Source: CAD feature listing. Evaluate the final solid. Frame: model axes, mm. Face numbers are marked on the shaded views. A direction names the side the tool comes from. Give positions to 0.01 mm unless a question says otherwise; leave off trailing zeros. Write each loop counter-clockwise with the first axis right and the second up, starting at its lowest first coordinate (ties: lowest second). Pieces come first, ordered by that corner, then holes. Notation, with made-up numbers: M 26,37.25 L 30,37.25 A15 ccw 30,41.25 Z; hole C 59.5,-1.5 d5. An arc over 180 degrees is marked long. Answer as a JSON object with one key per item and string values. Group by question number.
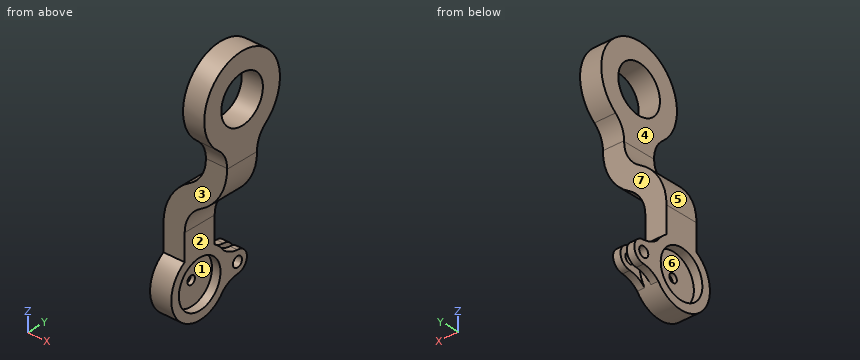
```python
from build123d import *

# Parameters (mm, degrees)
CROQUIS2_W              = 10
CROQUIS2_H              = 15.834903248
CROQUIS4_R              = 15
SALIENTE_EXTRUIR1_DEPTH = 10
CROQUIS5_R              = 20
SALIENTE_EXTRUIR2_DEPTH = 10
SALIENTE_EXTRUIR5_DEPTH = 3.5
CROQUIS13_R             = 2.4
CORTAR_EXTRUIR1_DEPTH   = 10
CROQUIS7_R              = 11
CORTAR_EXTRUIR3_DEPTH   = 10
REDONDEO2_R             = 12
REDONDEO3_R             = 12
CROQUIS14_R             = 11
CORTAR_EXTRUIR4_DEPTH   = 4
CROQUIS6_R              = 2
CORTAR_EXTRUIR5_DEPTH   = 6
CORTAR_EXTRUIR6_START   = -4
CROQUIS15_R             = 11
CORTAR_EXTRUIR6_DEPTH   = 4


with BuildPart() as part:
    # Barrer1: sweep along a path in Croquis1
    with BuildLine(Plane(origin=(0, 0, 0), x_dir=(1, 0, 0), z_dir=(0, 1, 0))) as barrer1_path:
        Line((-20, 85), (-20, 60))
        ThreePointArc((-20, 60), (-17.320508076, 50), (-10, 42.679491924))
        ThreePointArc((-10, 42.679491924), (-2.679491924, 35.358983849), (0, 25.358983849))
        Line((0, 25.358983849), (0, 0))
    # Croquis2 → Barrer1 (sweep)
    with BuildSketch(Plane.XY):
        Rectangle(CROQUIS2_W, CROQUIS2_H)
    sweep(path=barrer1_path.line)

    # Croquis4 → Saliente-Extruir1 (add)
    with BuildSketch(Plane(origin=(-15, 0, 0), x_dir=(0, 0, -1), z_dir=(1, 0, 0))):
        with Locations((85, 0)):
            Circle(CROQUIS4_R)
    extrude(amount=-SALIENTE_EXTRUIR1_DEPTH)

    # Croquis5 → Saliente-Extruir2 (add)
    with BuildSketch(Plane(origin=(5, 0, 0), x_dir=(0, 0, -1), z_dir=(1, 0, 0))):
        Circle(CROQUIS5_R)
    extrude(amount=-SALIENTE_EXTRUIR2_DEPTH)

    # Croquis12 → Saliente-Extruir5 (add)
    with BuildSketch(Plane(origin=(-15, 0, 0), x_dir=(0, 0, -1), z_dir=(1, 0, 0))):
        with BuildLine():
            ThreePointArc((90.068496439, 19.972615481), (85.068496439, 24.972615481), (80.068496439, 19.972615481))
            add(Edge.make_bspline(
                [(80.068496439, 19.972615481), (79.566731031, 15.028252388), (75.848465439, 11.643922813)],
                knots=[0, 0, 0, 1, 1, 1], degree=2))
            ThreePointArc((75.848465439, 11.643922813), (85.068496439, 14.846363713), (94.288527439, 11.643922813))
            add(Edge.make_bspline(
                [(90.068496439, 19.972615481), (90.570261847, 15.028252388), (94.288527439, 11.643922813)],
                knots=[0, 0, 0, 1, 1, 1], degree=2))
        make_face()
    saliente_extruir5 = extrude(amount=-SALIENTE_EXTRUIR5_DEPTH)

    # Simetría1: Saliente-Extruir5 across plane
    add(saliente_extruir5.mirror(Plane(origin=(-20, 0, 0), x_dir=(0, 0, 1), z_dir=(1, 0, 0))))

    # Croquis13 → Cortar-Extruir1 (cut)
    with BuildSketch(Plane(origin=(-15, 0, 0), x_dir=(0, 0, -1), z_dir=(1, 0, 0))):
        with Locations((85.068496439, 19.972615481)):
            Circle(CROQUIS13_R)
    extrude(amount=-CORTAR_EXTRUIR1_DEPTH, mode=Mode.SUBTRACT)

    # Croquis7 → Cortar-Extruir3 (cut)
    with BuildSketch(Plane(origin=(5, 0, 0), x_dir=(0, 0, -1), z_dir=(1, 0, 0))):
        Circle(CROQUIS7_R)
    extrude(amount=-CORTAR_EXTRUIR3_DEPTH, mode=Mode.SUBTRACT)

    # Redondeo2
    redondeo2_edges = [part.edges().sort_by_distance(p)[0] for p in [
        (0, 7.917451624, -18.366108999),
    ]]
    fillet(redondeo2_edges, radius=REDONDEO2_R)

    # Redondeo3
    redondeo3_edges = [part.edges().sort_by_distance(p)[0] for p in [
        (0, -7.917451624, -18.366108999),
    ]]
    fillet(redondeo3_edges, radius=REDONDEO3_R)

    # Croquis14 → Cortar-Extruir4 (cut)
    with BuildSketch(Plane.ZY.offset(25)):
        with Locations((-85, 0)):
            Circle(CROQUIS14_R)
    extrude(amount=-CORTAR_EXTRUIR4_DEPTH, mode=Mode.SUBTRACT)

    # Croquis6 → Cortar-Extruir5 (cut)
    with BuildSketch(Plane(origin=(-15, 0, 0), x_dir=(0, 0, -1), z_dir=(1, 0, 0))):
        with Locations((85, 0)):
            Circle(CROQUIS6_R)
    extrude(amount=-CORTAR_EXTRUIR5_DEPTH, mode=Mode.SUBTRACT)

    # Croquis15 → Cortar-Extruir6 (cut)
    with BuildSketch(Plane(origin=(-15, 0, 0), x_dir=(0, 0, -1), z_dir=(1, 0, 0)).offset(CORTAR_EXTRUIR6_START)):
        with Locations(Location((85, 0, 0), (0, 0, 180))):
            Circle(CROQUIS15_R)
    extrude(amount=CORTAR_EXTRUIR6_DEPTH, mode=Mode.SUBTRACT)


solid = part.part
```
(1) Section B-B, the plane y = 4. Return loops of the section in (x, z), plus the area to 3 significant figures.
(2) Section D-D, the plane y = 9. Return loops of the section in (x, z).
(3) Section C-C, the plane x = -3. Return loops of the section in (y, z), plus the area to 3 significant figures.
(4) Pull-direction query (Z, two-part tool) for the marked faces 5, 6 and 7; classes: pulls with the +Z half, pulls with the -Z half, needs draft (parallel to the pull), parting line crosses it, or undercut.
(5) Section A-A, the plane z = 0. Return loops of the section in (x, y).
(6) Ray query, L1, parallel to X at y = 11.5, z = -91.5; L2, parallel to Z at x = -0.5, y = 7.5; L3, parallel to Y at x = -11, z = -42.5. Return the intervals inside material, ascending. Write a range as [from, to].
(7) Access query for the marked faces 1, 2, 3 and 4. Directions: +Z, -Z, +X, -X, +Y, -Y. A direction counts if a zero-diameter tool reaches every point of the face in a straight line with its end or side. Return the directions, or none.
(8) Contact query for flat-ended pins moving along their axis: pin 1 Ø10 at (y, z) = (-8, -81) entering from -X; pin 2 Ø13 at (y, z) = (0, -85) entering from +X; pin 3 Ø1 at (x, z) = (-15, -42.5) entering from -Y; pin 4 Ø20 at (y, z) = (0, -1.5) entering from -X. Output: stop coordinate, or through.
Reported:
{
 "1": {"outline": "M -25,-99.46 L -15,-99.46 L -15,-95.25 L -19,-95.25 L -19,-74.75 L -15,-74.75 L -15,-60 A15 cw -7.5,-47.01 A25 ccw 5,-25.36 L 5,-10.25 L -5,-10.25 L -5,-25.36 A15 cw -12.5,-38.35 A25 ccw -25,-60 L -25,-74.75 L -21,-74.75 L -21,-95.25 L -25,-95.25 Z; M -5,10.25 L 5,10.25 L 5,19.6 L -5,19.6 Z", "area": "894 mm2"},
 "2": {"outline": "M -25,-97 L -15,-97 L -15,-91.32 L -19,-91.32 L -19,-78.68 L -15,-78.68 L -15,-73 L -25,-73 L -25,-78.68 L -21,-78.68 L -21,-91.32 L -25,-91.32 Z; M -5,-20.06 L 5,-20.06 L 5,-6.32 L -5,-6.32 Z; M -5,6.32 L 5,6.32 L 5,17.86 L -5,17.86 Z"},
 "3": {"outline": "M -12.45,-15.65 A12 cw -7.92,-25.05 L -7.92,-43.69 L 7.92,-43.69 L 7.92,-25.05 A12 cw 12.45,-15.65 A20 ccw long Z; hole C 0,0 d22", "area": "1,270 mm2"},
 "4": {"face 5": "pulls with the +Z half", "face 6": "undercut", "face 7": "needs draft"},
 "5": {"outline": "M -5,-20 L 5,-20 L 5,-11 L -5,-11 Z; M -5,11 L 5,11 L 5,20 L -5,20 Z"},
 "6": {"L1": "x = [-25, -15]", "L2": "z = [-41, -8.05], [8.05, 18.54]", "L3": "y = [-7.92, 7.92]"},
 "7": {"face 1": "+X", "face 2": "-Z, +X, +Y, -Y", "face 3": "+X, -X, -Y", "face 4": "+Z, -X, +Y, -Y"},
 "8": {"pin 1": "stops at x = -25", "pin 2": "stops at x = -19", "pin 3": "stops at y = -7.92", "pin 4": "stops at x = -5"}
}
